The listing builds one solid part. Answer for the finished solid, in the listing's coordinates (mm). A direction names the side the tool comes from. Round coordinates to 2 decimals unless told otherwise and drop trailing zeros. Order: outer loops, then holes, each group sorted by start corner. A loop starts at its lowest first (then second) coordinate and runs counter-clockwise, first axis right, second up. Notation, with made-up numbers: (57.5, 53.5) -> (76.5, 53.5) arc R26 ccw to (76.5, 80.5) -> close; hole circle Ø3 at (11.5, 59.5). An arc over 180 degrees is marked (long way). Answer in a Markdown table with one row per item. Add a question column.
```python
from build123d import *

# Parameters (mm, degrees)
SKETCH1_R           = 5.49275
BOSS_EXTRUDE1_DEPTH = 49.53
SKETCH2_R           = 2.3495
BOSS_EXTRUDE2_DEPTH = 45.72
CHAMFER1_SIZE       = 4.445
SKETCH3_R           = 2.8321
BOSS_EXTRUDE3_DEPTH = 3.2385


with BuildPart() as part:
    # Sketch1 → Boss-Extrude1 (new body)
    with BuildSketch(Plane.XY):
        Circle(SKETCH1_R)
    extrude(amount=BOSS_EXTRUDE1_DEPTH)

    # Sketch2 → Boss-Extrude2 (add)
    with BuildSketch(Plane.XY.offset(49.53)):
        Circle(SKETCH2_R)
    extrude(amount=BOSS_EXTRUDE2_DEPTH)

    # Chamfer1
    # the kernel refuses this chamfer: 4.445 mm, written as the material it takes off along each edge
    with BuildSketch(Plane(origin=(0, 0, 49.53), x_dir=(1, 0, 0), z_dir=(0, -1, 0))) as chamfer1_piece_1_section:
        Polygon((5.49275, -CHAMFER1_SIZE), (5.49275 - CHAMFER1_SIZE, 0), (5.49275, 0), align=None)
    chamfer1_piece_1 = revolve(axis=Axis((0, 0, 49.53), (0, 0, 1)), mode=Mode.PRIVATE)
    chamfer1_piece_1 = chamfer1_piece_1 - Plane(origin=(0, 0, 46.639044466), x_dir=(1, 0, 0), z_dir=(0, 0, -1)) * Cylinder(2.3495, 22, mode=Mode.PRIVATE)
    add(chamfer1_piece_1, mode=Mode.SUBTRACT)

    # Sketch3 → Boss-Extrude3 (add)
    with BuildSketch(Plane(origin=(0, 0, 0), x_dir=(-1, 0, 0), z_dir=(0, 0, -1))):
        Circle(SKETCH3_R)
    extrude(amount=BOSS_EXTRUDE3_DEPTH)


solid = part.part
```
1. The part is cut by section C-C (z = 18.5). Give the vertices of the cut face in (x, y), then the cut area to 3 significant figures.
2. The part is cut by section D-D (z = 87.5). Give the vertices of the cut face in (x, y), then the cut area to 3 significant figures.
3. The mould has two halves that part along X. Classify faces 4 (the flat face through (-1, 3, 0)), 5 (the conical face through (1.15, -2.22, 48.08)): released by +X, released by -X, zero draft, split by the parting line, or undercut.
4. Straight lines are drawn through the part: line 1 along X through (y, z) = (0, 67.5); line 2 along Z through (x, y) = (1.5, 5); line 3 along Z through (x, y) = (-2, -4.5). For each, find the intervals that lie inside material, in ascending order.
5. Each of these flat-tipped pins is pushed along its axis until it touches: pin 1 (2 mm diameter, centred on x = 0, z = 77.5, fed in from -Y); pin 2 (1 mm diameter, centred on x = 1.5, z = 17.5, fed in from +Y); pin 3 (6 mm diameter, centred on x = 4, z = 28, fed in from -Y); pin 4 (2 mm diameter, centred on x = -4.5, z = 64.5, fed in from +Y). Where does it stop, or does it pass through?
6. For faces 1 (the flat face through (0, 0, 95.25)), 2 (the cylindrical face through (-0.31, -2.33, 71.41)), 3 (the cylindrical face through (2.25, -1.72, -1.6)), determine the directions among +Z, -Z, +X, -X, +Y, -Y from which every point of the face is accessible in a straight line to the end or side of a thin tool.
Report:
| question | item | result |
|---|---|---|
| 1 | outline | circle Ø10.99 at (0, 0) |
| 1 | area | 94.8 mm^2 |
| 2 | outline | circle Ø4.7 at (0, 0) |
| 2 | area | 17.3 mm^2 |
| 3 | face 4 | zero draft |
| 3 | face 5 | split by the parting line |
| 4 | line 1 | x = -2.35 to 2.35 |
| 4 | line 2 | z = 0 to 45.36 |
| 4 | line 3 | z = 0 to 45.65 |
| 5 | pin 1 | stops at y = -2.35 |
| 5 | pin 2 | stops at y = 5.4 |
| 5 | pin 3 | stops at y = -5.4 |
| 5 | pin 4 | passes through |
| 6 | face 1 | +Z, +X, -X, +Y, -Y |
| 6 | face 2 | +Z |
| 6 | face 3 | -Z |
